```python
from build123d import *

# Parameters (mm, degrees)
SKETCH1_R           = 42.5
BOSS_EXTRUDE1_DEPTH = 17
CUT_EXTRUDE3_DEPTH  = 17
SKETCH4_R           = 5.1
CUT_EXTRUDE4_DEPTH  = 17
SKETCH5_R           = 6
SKETCH5_R_2         = 5.1
BOSS_EXTRUDE2_DEPTH = 4
SKETCH6_R           = 6
SKETCH6_R_2         = 5.1
BOSS_EXTRUDE3_DEPTH = 4
FILLET1_R           = 5
FILLET2_R           = 5


with BuildPart() as part:
    # Sketch1 → Boss-Extrude1 (new body)
    with BuildSketch(Plane.XY):
        Circle(SKETCH1_R)
    extrude(amount=BOSS_EXTRUDE1_DEPTH)

    # Sketch3 → Cut-Extrude3 (cut)
    with BuildSketch(Plane.XY.offset(17)):
        with BuildLine():
            ThreePointArc((-8.711670849, 4.9098667), (-6.128694511, 7.901841785), (-2.588190451, 9.659258263))
            Line((-2.588190451, 9.659258263), (-7.893980876, 29.460737702))
            ThreePointArc((-7.893980876, 29.460737702), (-18.692518258, 24.100617444), (-26.570596091, 14.975093435))
            Line((-26.570596091, 14.975093435), (-8.711670849, 4.9098667))
        make_face()
        with BuildLine():
            Line((7.893980876, 29.460737702), (2.588190451, 9.659258263))
            ThreePointArc((2.588190451, 9.659258263), (5.877852523, 8.090169944), (8.386705679, 5.44639035))
            Line((8.386705679, 5.44639035), (25.579452322, 16.611490568))
            ThreePointArc((25.579452322, 16.611490568), (17.927450195, 24.675018328), (7.893980876, 29.460737702))
        make_face()
        with BuildLine():
            Line((30.45820081, 1.596246665), (9.986295348, 0.523359562))
            ThreePointArc((9.986295348, 0.523359562), (9.99657325, 0.261769483), (10, 0))
            ThreePointArc((10, 0), (9.426414911, -3.338068592), (7.771459615, -6.29320391))
            Line((7.771459615, -6.29320391), (23.702951824, -19.194271927))
            ThreePointArc((23.702951824, -19.194271927), (28.750565478, -10.181109207), (30.5, 0))
            ThreePointArc((30.5, 0), (30.489548412, 0.798396923), (30.45820081, 1.596246665))
        make_face()
        with BuildLine():
            Line((10.930222461, -28.474203008), (3.583679495, -9.335804265))
            ThreePointArc((3.583679495, -9.335804265), (0, -10), (-3.583679495, -9.335804265))
            Line((-3.583679495, -9.335804265), (-10.930222461, -28.474203008))
            ThreePointArc((-10.930222461, -28.474203008), (0, -30.5), (10.930222461, -28.474203008))
        make_face()
        with BuildLine():
            Line((-23.702951824, -19.194271927), (-7.771459615, -6.29320391))
            ThreePointArc((-7.771459615, -6.29320391), (-9.510565163, -3.090169944), (-9.986295348, 0.523359562))
            Line((-9.986295348, 0.523359562), (-30.45820081, 1.596246665))
            ThreePointArc((-30.45820081, 1.596246665), (-29.007223747, -9.425018328), (-23.702951824, -19.194271927))
        make_face()
    extrude(amount=-CUT_EXTRUDE3_DEPTH, mode=Mode.SUBTRACT)

    # Sketch4 → Cut-Extrude4 (cut)
    with BuildSketch(Plane.XY.offset(17)):
        Circle(SKETCH4_R)
    extrude(amount=-CUT_EXTRUDE4_DEPTH, mode=Mode.SUBTRACT)

    # Sketch5 → Boss-Extrude2 (add)
    with BuildSketch(Plane.XY.offset(17)):
        Circle(SKETCH5_R)
        Circle(SKETCH5_R_2, mode=Mode.SUBTRACT)
    extrude(amount=BOSS_EXTRUDE2_DEPTH)

    # Sketch6 → Boss-Extrude3 (add)
    with BuildSketch(Plane(origin=(0, 0, 0), x_dir=(-1, 0, 0), z_dir=(0, 0, -1))):
        Circle(SKETCH6_R)
        Circle(SKETCH6_R_2, mode=Mode.SUBTRACT)
    extrude(amount=BOSS_EXTRUDE3_DEPTH)

    # Sketch10 → Cut-Revolve1 (revolve, cut)
    with BuildSketch(Plane(origin=(0, 0, 0), x_dir=(0, 0, -1), z_dir=(1, 0, 0))):
        Polygon((-16, 42.5), (-8.5, 42.5), (-8.5, 37.459040498), (-12, 37.459040498), align=None)
        Polygon((-8.5, 42.5), (-1, 42.5), (-5, 37.459040498), (-8.5, 37.459040498), align=None)
    revolve(axis=Axis((0, 0, 0), (0, 0, -1)), mode=Mode.SUBTRACT)

    # Fillet1
    fillet1_edges = [part.edges().sort_by_distance(p)[0] for p in [
        (0, -37.459040498, 5),
    ]]
    fillet(fillet1_edges, radius=FILLET1_R)

    # Fillet2
    fillet2_edges = [part.edges().sort_by_distance(p)[0] for p in [
        (0, -37.459040498, 12),
    ]]
    fillet(fillet2_edges, radius=FILLET2_R)


solid = part.part
```
Build history of the part. All positions in model axes, mm. A direction names the side the tool comes from. Give positions to 0.01 mm unless a question says otherwise; leave off trailing zeros. Loops run counter-clockwise (first coordinate to the right, second up) from the corner with the lowest first, then second, coordinate; pieces in that order, holes last. Notation, with made-up numbers: (-28.5, 23.5) -> (-11.5, 23.5) arc R7 cw to (-11.5, 30.5) -> close; hole circle Ø7 at (-9.5, 84.5). An arc over 180 degrees is marked (long way). One line per question, with ' | ' between items.
Q1. Drop flat-ended pins along their axis: pin 1 (1.5 mm diameter, centred on x = -20, y = -33, fed in from +Z); pin 2 (6 mm diameter, centred on y = -9.5, z = 12.5, fed in from +X); pin 3 (12 mm diameter, centred on x = -29, y = 31.5, fed in from -Z). Give the stop position or say it passes through.
Filled sheet:
pin 1: stops at z = 17 | pin 2: stops at x = 40.84 | pin 3: stops at z = 0
Q2. Drill centre lines: line 1 along Y through (x, z) = (0, -1.4); line 2 along X through (y, z) = (19, 2.75); line 3 along Y through (x, z) = (11, 14.75). Where is each one in solid material? Low to high. Write a range as [from, to].
Filled sheet:
line 1: y = [-6, -5.1], [5.1, 6] | line 2: x = [-35.53, -23.86], [-5.09, 5.09], [23.86, 35.53] | line 3: y = [-39.42, -8.91], [0.58, 7.14], [28.45, 39.42]
Q3. Pull direction Y, two halves, no side cores. Call faces 5 (the cylindrical face through (-29.055, -9.276, 8.619)), 6 (the cylindrical face through (6, 8, 9)), 7 (the cylindrical face through (40.537, 12.766, 16.493)), 8 (the flat face through (9, 1, 17)): pulls with the +Y half, pulls with the -Y half, needs draft (parallel to the pull), parting line crosses it, or undercut.
Filled sheet:
face 5: undercut | face 6: undercut | face 7: parting line crosses it | face 8: needs draft
Q4. Cut at A-A, the plane x = 0. Count the separate pieces of the cut face and the enclosed holes in it, plus the area to 3 significant figures.
Filled sheet:
separate pieces: 3 | enclosed holes: 0 | area: 830 mm²
Q5. Cut at B-B, the plane z = 18. Write the cut outline in (x, y), plus the area to 3 significant figures.
Filled sheet:
outline: circle Ø12 at (0, 0); hole circle Ø10.2 at (0, 0) | area: 31.4 mm²
Q6. Tool access for faces 1 (the cylindrical face through (-6, 0, 19)), 2 (the cylindrical face through (-0.2, -30.5, 8.6)), 3 (the conical face through (39.168, -5.143, 3.377)), 4 (the cylindrical face through (6, 0, -2)): list every direction of +Z, -Z, +X, -X, +Y, -Y with a clear straight run to the whole face (end or side of a thin tool).
Filled sheet:
face 1: +Z | face 2: +Z, -Z | face 3: none | face 4: -Z
